Source: CAD feature listing. Evaluate the final solid. Frame: model axes, mm. Face numbers are marked on the shaded views. A direction names the side the tool comes from. Coordinates: 2 decimals unless noted, no trailing zeros. Order: outer loops, then holes, each group sorted by start corner. A loop starts at its lowest first (then second) coordinate and runs counter-clockwise, first axis right, second up. Notation, with made-up numbers: (36.5, 47) - (91.5, 47) arc R19 ccw to (91.5, 62) - close; hole circle Ø5 at (-22, -4). An arc over 180 degrees is marked (long way). One line per question, with ' | ' between items.
from build123d import *

# Parameters (mm, degrees)
SCHIZZO1_W                    = 20
SCHIZZO1_H                    = 20
ESTRUSIONE_ESTRUSIONE1_DEPTH  = 58.2
SCHIZZO2_R                    = 3
TAGLIO_ESTRUSIONE1_DEPTH      = 60.893572276
FORO_FILETTATO_G1_8_1_D       = 8.8
FORO_FILETTATO_G1_8_1_DEPTH   = 10
FORO_FILETTATO_G1_8_1_TIP     = 2.643786724
TAGLIO_ESTRUSIONE5_DEPTH      = 63.347734522
TAGLIO_ESTRUSIONE5_DEPTH_BACK = 63.347734522
FORO_FILETTATO_M3_1_D         = 2.5
FORO_FILETTATO_M3_1_DEPTH     = 5
FORO_FILETTATO_M3_1_TIP       = 0.751075774
FORO_FILETTATO_M3_2_D         = 2.5
M4_CLEARANCE_HOLE1_D          = 5


with BuildPart() as part:
    # Schizzo1 → Estrusione-Estrusione1 (new body)
    with BuildSketch(Plane.XY):
        Rectangle(SCHIZZO1_W, SCHIZZO1_H)
    extrude(amount=-ESTRUSIONE_ESTRUSIONE1_DEPTH)

    # Schizzo2 → Taglio-Estrusione1 (cut, through all)
    with BuildSketch(Plane(origin=(0, 0, -58.2), x_dir=(-1, 0, 0), z_dir=(0, 0, -1))):
        Circle(SCHIZZO2_R)
    extrude(amount=-TAGLIO_ESTRUSIONE1_DEPTH, mode=Mode.SUBTRACT)

    # Foro filettato G1/8-1
    with Locations(Plane.XY):
        with Locations((0, 0)):
            Hole(FORO_FILETTATO_G1_8_1_D / 2, depth=FORO_FILETTATO_G1_8_1_DEPTH)
            with Locations((0, 0, -(FORO_FILETTATO_G1_8_1_DEPTH + FORO_FILETTATO_G1_8_1_TIP / 2))):  # 118° drill point
                Cone(0, FORO_FILETTATO_G1_8_1_D / 2, FORO_FILETTATO_G1_8_1_TIP, mode=Mode.SUBTRACT)

    # Schizzo10 → Taglio-Estrusione5 (cut, two sides: drawn at the far end of the back side and taken through both)
    with BuildSketch(Plane(origin=(10, 0, 0), x_dir=(0, 0, -1), z_dir=(1, 0, 0)).offset(-TAGLIO_ESTRUSIONE5_DEPTH_BACK)):
        Polygon((-131.2640095, -7), (0, -7), (46, -7), (46, -10), (46, -141.2640095), (-112.509379382, -350.53832089), (-289.773388882, -216.27431139), align=None)
    extrude(amount=TAGLIO_ESTRUSIONE5_DEPTH + TAGLIO_ESTRUSIONE5_DEPTH_BACK, mode=Mode.SUBTRACT)

    # Foro filettato M3-1
    with Locations(Plane(origin=(0, 10, -29.1), x_dir=(1, 0, 0), z_dir=(0, 1, 0))):
        with Locations((0, 0)):
            Hole(FORO_FILETTATO_M3_1_D / 2, depth=FORO_FILETTATO_M3_1_DEPTH)
            with Locations((0, 0, -(FORO_FILETTATO_M3_1_DEPTH + FORO_FILETTATO_M3_1_TIP / 2))):  # 118° drill point
                Cone(0, FORO_FILETTATO_M3_1_D / 2, FORO_FILETTATO_M3_1_TIP, mode=Mode.SUBTRACT)

    # Schizzo14 → Foro Ø16.0 (16)-1 (revolve, cut)
    with BuildSketch(Plane(origin=(0, 0, -58.2), x_dir=(0, 1, 0), z_dir=(1, 0, 0))):
        Polygon((0, 0), (0, 16.806884952), (8, 12), (8, 0), align=None)
    revolve(axis=Axis((0, 0, -64.55), (0, 0, 1)), mode=Mode.SUBTRACT)

    # Foro filettato M3-2 (through all)
    with Locations(Plane(origin=(10, 5.5, -53.2), x_dir=(0, 0, 1), z_dir=(1, 0, 0))):
        with Locations((0, 0), (0, 11)):
            Hole(FORO_FILETTATO_M3_2_D / 2)

    # M4 Clearance Hole1 (through all)
    with Locations(Plane(origin=(10, 6, -19.1), x_dir=(0, 0, 1), z_dir=(1, 0, 0))):
        with Locations((0, 0), (-20, 0)):
            Hole(M4_CLEARANCE_HOLE1_D / 2)


solid = part.part
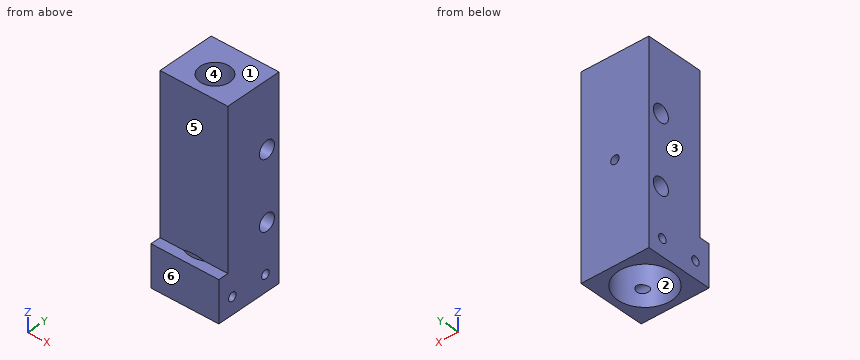
(1) Cut plane C-C (z = -53.2). Return the cut outline in (x, y), and give its area (3 significant figures).
Taken from the geometry:
outline: (-10, -10) - (10, -10) - (10, -6.75) - (4.29, -6.75) arc R8 cw to (-4.29, -6.75) - (-10, -6.75) - close; (-10, -4.25) - (-6.78, -4.25) arc R8 cw to (-6.78, 4.25) - (-10, 4.25) - close; (-10, 6.75) - (-4.29, 6.75) arc R8 cw to (4.29, 6.75) - (10, 6.75) - (10, 10) - (-10, 10) - close; (6.78, -4.25) - (10, -4.25) - (10, 4.25) - (6.78, 4.25) arc R8 cw to start | area: 156 mm²
(2) Pin query (flat end, axial travel): P1, Ø12, axis at x = -2.5, y = 2, coming from the +Z side; P2, Ø1.5, axis at x = 3, y = -9, coming from the +Z side; P3, Ø2, axis at y = -5.5, z = -53.2, coming from the -X side; P4, Ø8, axis at x = -1, z = -6.5, coming from the -Y side. Return the tip coordinate at first contact, or that it passes through.
Taken from the geometry:
P1: stops at z = 0 | P2: stops at z = -46 | P3: passes through | P4: stops at y = -7
(3) Set-up query: the marked faces 4, 5 and 6. Return all of +Z, -Z, +X, -X, +Y, -Y with unobstructed straight access to the full face (end or side cutting, diameter ignored); none if empty.
Taken from the geometry:
face 4: +Z | face 5: +Z, +X, -X, -Y | face 6: +Z, -Z, +X, -X, -Y
(4) Pull-direction query (X, two-part tool) for the marked faces 1, 2 and 3; classes: pulls with the +X half, pulls with the -X half, needs draft (parallel to the pull), parting line crosses it, or undercut.
Taken from the geometry:
face 1: needs draft | face 2: undercut | face 3: pulls with the -X half
(5) Cut plane A-A (z = -19.1). Return the cut outline in (x, y), and give its area (3 significant figures).
Taken from the geometry:
outline: (-10, -7) - (10, -7) - (10, 3.5) - (-10, 3.5) - close; (-10, 8.5) - (10, 8.5) - (10, 10) - (-10, 10) - close; hole circle Ø6 at (0, 0) | area: 212 mm²
(6) Cut plane B-B (z = -4.5). Return the cut outline in (x, y), and give its area (3 significant figures).
Taken from the geometry:
outline: (-10, -7) - (10, -7) - (10, 10) - (-10, 10) - close; hole circle Ø8.8 at (0, 0) | area: 279 mm²
(7) Material intervals for L1, parallel to Y at x = -1.25, z = -39; L2, parallel to X at y = 0, z = -52.75; L3, parallel to Z at x = 0, y = 6.35, sorted ascending. Write a range as from..to.
Taken from the geometry:
L1: y = -7..-2.73, 2.73..3.5, 8.5..10 | L2: x = -10..-8, 8..10 | L3: z = -45.21..-41.58, -36.62..-30.35, -27.85..-21.58, -16.62..0
(8) Cut plane D-D (x = 2.25). State how many separate pieces and enclosed holes the cut face has, and give its area (3 significant figures).
Taken from the geometry:
separate pieces: 3 | enclosed holes: 2 | area: 564 mm²
